from build123d import *

# Parameters (mm, degrees)
F0_R     = 6
F1_DEPTH = 15
F2_R     = 9.45


with BuildPart() as f1:
    # F0 (on Top) → F1 (new body)
    with BuildSketch(Plane.XY):
        with BuildLine():
            Line((12.517717, -2.227194), (9.759653, -1.331044))
            ThreePointArc((9.759653, -1.331044), (9.367907, -3.043817), (8.678093, -4.659742))
            Line((8.678093, -4.659742), (11.436157, -5.555892))
            Line((11.436157, -5.555892), (13.647287, -5.222869))
            Line((13.647287, -5.222869), (14.110813, -3.796284))
            Line((14.110813, -3.796284), (12.517717, -2.227194))
        make_face()
        with BuildLine():
            Line((8.817934, -9.159567), (7.113357, -6.813418))
            ThreePointArc((7.113357, -6.813418), (5.789685, -7.968817), (4.281797, -8.870666))
            Line((4.281797, -8.870666), (5.986374, -11.216815))
            Line((5.986374, -11.216815), (7.970962, -12.247064))
            Line((7.970962, -12.247064), (9.184487, -11.365386))
            Line((9.184487, -11.365386), (8.817934, -9.159567))
        make_face()
        with BuildLine():
            ThreePointArc((9.759653, -1.331044), (9.827387, -0.667054), (9.85, 0))
            ThreePointArc((9.85, 0), (9.827387, 0.667054), (9.759653, 1.331044))
            ThreePointArc((9.759653, 1.331044), (9.367907, 3.043817), (8.678093, 4.659742))
            ThreePointArc((8.678093, 4.659742), (7.968817, 5.789685), (7.113357, 6.813418))
            ThreePointArc((7.113357, 6.813418), (5.789685, 7.968817), (4.281797, 8.870666))
            ThreePointArc((4.281797, 8.870666), (3.043817, 9.367907), (1.75, 9.693297))
            ThreePointArc((1.75, 9.693297), (0, 9.85), (-1.75, 9.693297))
            ThreePointArc((-1.75, 9.693297), (-3.043817, 9.367907), (-4.281797, 8.870666))
            ThreePointArc((-4.281797, 8.870666), (-5.789685, 7.968817), (-7.113357, 6.813418))
            ThreePointArc((-7.113357, 6.813418), (-7.968817, 5.789685), (-8.678093, 4.659742))
            ThreePointArc((-8.678093, 4.659742), (-9.367907, 3.043817), (-9.759653, 1.331044))
            ThreePointArc((-9.759653, 1.331044), (-9.85, 0), (-9.759653, -1.331044))
            ThreePointArc((-9.759653, -1.331044), (-9.367907, -3.043817), (-8.678093, -4.659742))
            ThreePointArc((-8.678093, -4.659742), (-7.968817, -5.789685), (-7.113357, -6.813418))
            ThreePointArc((-7.113357, -6.813418), (-5.789685, -7.968817), (-4.281797, -8.870666))
            ThreePointArc((-4.281797, -8.870666), (-3.043817, -9.367907), (-1.75, -9.693297))
            ThreePointArc((-1.75, -9.693297), (0, -9.85), (1.75, -9.693297))
            ThreePointArc((1.75, -9.693297), (3.043817, -9.367907), (4.281797, -8.870666))
            ThreePointArc((4.281797, -8.870666), (5.789685, -7.968817), (7.113357, -6.813418))
            ThreePointArc((7.113357, -6.813418), (7.968817, -5.789685), (8.678093, -4.659742))
            ThreePointArc((8.678093, -4.659742), (9.367907, -3.043817), (9.759653, -1.331044))
        make_face()
        Circle(F0_R, mode=Mode.SUBTRACT)
        with BuildLine():
            ThreePointArc((8.678093, 4.659742), (9.367907, 3.043817), (9.759653, 1.331044))
            Line((9.759653, 1.331044), (12.517717, 2.227194))
            Line((12.517717, 2.227194), (14.110813, 3.796284))
            Line((14.110813, 3.796284), (13.647287, 5.222869))
            Line((13.647287, 5.222869), (11.436157, 5.555892))
            Line((11.436157, 5.555892), (8.678093, 4.659742))
        make_face()
        with BuildLine():
            ThreePointArc((4.281797, 8.870666), (5.789685, 7.968817), (7.113357, 6.813418))
            Line((7.113357, 6.813418), (8.817934, 9.159567))
            Line((8.817934, 9.159567), (9.184487, 11.365386))
            Line((9.184487, 11.365386), (7.970962, 12.247064))
            Line((7.970962, 12.247064), (5.986374, 11.216815))
            Line((5.986374, 11.216815), (4.281797, 8.870666))
        make_face()
        with BuildLine():
            ThreePointArc((-1.75, 9.693297), (0, 9.85), (1.75, 9.693297))
            Line((1.75, 9.693297), (1.75, 12.593297))
            Line((1.75, 12.593297), (0.75, 14.593297))
            Line((0.75, 14.593297), (-0.75, 14.593297))
            Line((-0.75, 14.593297), (-1.75, 12.593297))
            Line((-1.75, 12.593297), (-1.75, 9.693297))
        make_face()
        with BuildLine():
            ThreePointArc((-7.113357, 6.813418), (-5.789685, 7.968817), (-4.281797, 8.870666))
            Line((-4.281797, 8.870666), (-5.986374, 11.216815))
            Line((-5.986374, 11.216815), (-7.970962, 12.247064))
            Line((-7.970962, 12.247064), (-9.184487, 11.365386))
            Line((-9.184487, 11.365386), (-8.817934, 9.159567))
            Line((-8.817934, 9.159567), (-7.113357, 6.813418))
        make_face()
        with BuildLine():
            ThreePointArc((-9.759653, 1.331044), (-9.367907, 3.043817), (-8.678093, 4.659742))
            Line((-8.678093, 4.659742), (-11.436157, 5.555892))
            Line((-11.436157, 5.555892), (-13.647287, 5.222869))
            Line((-13.647287, 5.222869), (-14.110813, 3.796284))
            Line((-14.110813, 3.796284), (-12.517717, 2.227194))
            Line((-12.517717, 2.227194), (-9.759653, 1.331044))
        make_face()
        with BuildLine():
            Line((-11.436157, -5.555892), (-8.678093, -4.659742))
            ThreePointArc((-8.678093, -4.659742), (-9.367907, -3.043817), (-9.759653, -1.331044))
            Line((-9.759653, -1.331044), (-12.517717, -2.227194))
            Line((-12.517717, -2.227194), (-14.110813, -3.796284))
            Line((-14.110813, -3.796284), (-13.647287, -5.222869))
            Line((-13.647287, -5.222869), (-11.436157, -5.555892))
        make_face()
        with BuildLine():
            Line((-5.986374, -11.216815), (-4.281797, -8.870666))
            ThreePointArc((-4.281797, -8.870666), (-5.789685, -7.968817), (-7.113357, -6.813418))
            Line((-7.113357, -6.813418), (-8.817934, -9.159567))
            Line((-8.817934, -9.159567), (-9.184487, -11.365386))
            Line((-9.184487, -11.365386), (-7.970962, -12.247064))
            Line((-7.970962, -12.247064), (-5.986374, -11.216815))
        make_face()
        with BuildLine():
            Line((1.75, -12.593297), (1.75, -9.693297))
            ThreePointArc((1.75, -9.693297), (0, -9.85), (-1.75, -9.693297))
            Line((-1.75, -9.693297), (-1.75, -12.593297))
            Line((-1.75, -12.593297), (-0.75, -14.593297))
            Line((-0.75, -14.593297), (0.75, -14.593297))
            Line((0.75, -14.593297), (1.75, -12.593297))
        make_face()
    extrude(amount=F1_DEPTH)

    # F2
    f2_edges = [f1.edges().sort_by_distance(p)[0] for p in [
        (8.817934, -9.159567, 7.5),
        (5.986374, -11.216815, 7.5),
        (11.436157, -5.555892, 7.5),
        (12.517717, -2.227194, 7.5),
        (12.517717, 2.227194, 7.5),
        (11.436157, 5.555892, 7.5),
        (8.817934, 9.159567, 7.5),
        (5.986374, 11.216815, 7.5),
        (1.75, 12.593297, 7.5),
        (-1.75, 12.593297, 7.5),
        (-5.986374, 11.216815, 7.5),
        (-8.817934, 9.159567, 7.5),
        (-11.436157, 5.555892, 7.5),
        (-12.517717, 2.227194, 7.5),
        (-12.517717, -2.227194, 7.5),
        (-11.436157, -5.555892, 7.5),
        (-8.817934, -9.159567, 7.5),
        (-5.986374, -11.216815, 7.5),
        (-1.75, -12.593297, 7.5),
        (1.75, -12.593297, 7.5),
    ]]
    fillet(f2_edges, radius=F2_R)


solid = f1.part
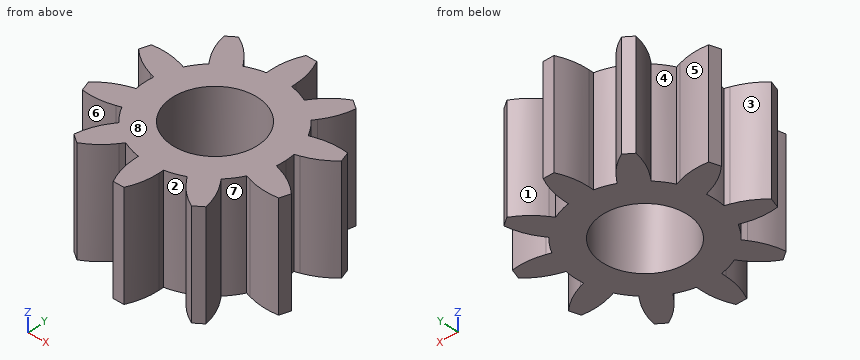
Model file for the job. Use its own axes, mm. Face numbers are marked on the shaded views. A direction names the side the tool comes from. Round coordinates to 2 decimals unless told otherwise and drop trailing zeros. Loops run counter-clockwise (first coordinate to the right, second up) from the corner with the lowest first, then second, coordinate; pieces in that order, holes last. Notation, with made-up numbers: M 11,-1 L 59,-1 A18 cw 59,14 Z; hole C -37,50 d3. An arc over 180 degrees is marked long. One line per question, with ' | ' between items.
1) Flat gauge pins, fed straight in: pin 1 (2 mm diameter, centred on x = -10.5, z = 3, fed in from -Y); pin 2 (2 mm diameter, centred on y = -10.5, z = 9, fed in from +X); pin 3 (12 mm diameter, centred on x = 3, y = 8, fed in from -Z); pin 4 (3 mm diameter, centred on y = 8, z = 2, fed in from -X) (3 decimals). Where does each tip first touch, or does it go through?
Solved:
pin 1: stops at y = -5.3 | pin 2: stops at x = 9.18 | pin 3: stops at z = 0 | pin 4: stops at x = -8.675
2) 3-axis set-ups, long thin cutter, end or side, ignore diameter. For the marked faces 1, 2, 3 and 4: which of +Z, -Z, +X, -X, +Y, -Y reach the whole face in a straight line?
Solved:
face 1: +Z, -Z, +Y | face 2: +Z, -Z, -Y | face 3: +Z, -Z, -X | face 4: +Z, -Z
3) Band-saw the part on B-B (y = 10.75). Give the cut face in (x, z), then the cut area to 3 significant figures.
Solved:
outline: M -9.06,0 L -5.86,0 L -5.86,15 L -9.06,15 Z; M -1.74,0 L 1.74,0 L 1.74,15 L -1.74,15 Z; M 5.86,0 L 9.06,0 L 9.06,15 L 5.86,15 Z | area: 148 mm²
4) Drill centre lines: line 1 along Y through (x, z) = (0, 8.75); line 2 along Y through (x, z) = (-8.5, 12.75); line 3 along Y through (x, z) = (8.25, 8.75). Where is each one in solid material? Low to high.
Solved:
line 1: y = -14.59 to -6, 6 to 14.59 | line 2: y = -11.86 to -9.08, -4.98 to 4.98, 9.08 to 11.86 | line 3: y = -12.04 to -8.56, -5.38 to 5.38, 8.56 to 12.04
5) Band-saw the part on C-C (y = -2.5). Give the cut face in (x, z).
Solved:
outline: M -12.47,0 L -5.45,0 L -5.45,15 L -12.47,15 Z; M 5.45,0 L 12.47,0 L 12.47,15 L 5.45,15 Z
6) Band-saw the part on A-A (x = 0). Give the cut face in (y, z), then the cut area to 3 significant figures.
Solved:
outline: M -14.59,0 L -6,0 L -6,15 L -14.59,15 Z; M 6,0 L 14.59,0 L 14.59,15 L 6,15 Z | area: 258 mm²
7) Mould opens along Y. For the marked faces 5, 6, 7 and 8 say: +Y half, -Y half, draft (parallel to the pull), parting line (faces both ways), or undercut.
Solved:
face 5: +Y half | face 6: -Y half | face 7: undercut | face 8: draft
8) Band-saw the part on D-D (y = -8.25). Give the cut face in (x, z).
Solved:
outline: M -8.08,0 L 8.08,0 L 8.08,15 L -8.08,15 Z
